```python
from build123d import *

# Parameters (mm, degrees)
SKETCH2_R                = 50.8
BOSS_EXTRUDE1_DEPTH      = 76.2
CUT_EXTRUDE4_START       = -6.35
SKETCH5_R                = 44.449999999999996
CUT_EXTRUDE4_DEPTH       = 63.5
CUT_EXTRUDE6_REACH       = 106.727
SKETCH14_R               = 7.62
BOSS_EXTRUDE4_REACH      = 170.227
BOSS_EXTRUDE4_END_RADIUS = 50.8
BOSS_EXTRUDE4_START      = 63.5
SKETCH17_W               = 52.06999999999999
SKETCH17_H               = 52.06999999999999
SKETCH15_W               = 11.430000000000003
SKETCH15_H               = 11.430000000000021
CUT_EXTRUDE7_DEPTH       = 112.44204771987995
CUT_EXTRUDE9_DEPTH       = 12.7
CUT_EXTRUDE10_DEPTH      = 112.44204771987995
CUT_EXTRUDE10_DEPTH_BACK = 112.44204771987995
SKETCH22_R               = 1.9049999999999998
SKETCH22_R_2             = 1.905
CUT_EXTRUDE11_DEPTH      = 6.35
CUT_EXTRUDE12_REACH      = 113.442
CUT_EXTRUDE12_END_RADIUS = 50.8


with BuildPart() as part:
    # Sketch2 → Boss-Extrude1 (new body)
    with BuildSketch(Plane(origin=(0, 0, 0), x_dir=(1, 0, 0), z_dir=(0, 1, 0))):
        with Locations(Location((0, 0, 0), (0, 0, 270))):
            Circle(SKETCH2_R)
    extrude(amount=-BOSS_EXTRUDE1_DEPTH)

    # Sketch5 → Cut-Extrude4 (cut)
    with BuildSketch(Plane(origin=(0, 0, 0), x_dir=(1, 0, 0), z_dir=(0, 1, 0)).offset(CUT_EXTRUDE4_START)):
        with Locations(Location((0, 0, 0), (0, 0, 270))):
            Circle(SKETCH5_R)
    extrude(amount=-CUT_EXTRUDE4_DEPTH, mode=Mode.SUBTRACT)

    # Sketch14 → Cut-Extrude6 (cut, up to next)
    with BuildSketch(Plane(origin=(0, 0, 0), x_dir=(1, 0, 0), z_dir=(0, 1, 0)), mode=Mode.PRIVATE) as cut_extrude6_sk1:
        with Locations(Location((0, 0, 0), (0, 0, 270))):
            Circle(SKETCH14_R)
    cut_extrude6_tool1 = extrude(cut_extrude6_sk1.sketch, amount=-CUT_EXTRUDE6_REACH, mode=Mode.PRIVATE) & part.part
    add(cut_extrude6_tool1.solids().sort_by_distance((0, 0, 0))[0], mode=Mode.SUBTRACT)

    # Boss-Extrude4: up to this cylinder (the profile starts outside it)
    boss_extrude4_end = Plane(origin=(0, -50.165, 0), z_dir=(0, 1, 0)) * Cylinder(BOSS_EXTRUDE4_END_RADIUS, 443.054, mode=Mode.PRIVATE)
    # Sketch17 → Boss-Extrude4 (add, up to the surface)
    with BuildSketch(Plane(origin=(0, 0, 0), x_dir=(0, 0, -1), z_dir=(1, 0, 0)).offset(BOSS_EXTRUDE4_START), mode=Mode.PRIVATE) as boss_extrude4_sk1:
        with Locations((0, -50.165000000000006)):
            Rectangle(SKETCH17_W, SKETCH17_H)
    boss_extrude4_tool1 = extrude(boss_extrude4_sk1.sketch, amount=-BOSS_EXTRUDE4_REACH, mode=Mode.PRIVATE) - boss_extrude4_end
    add(boss_extrude4_tool1.solids().sort_by_distance((63.5, -50.165, 0))[0])

    # Sketch15 → Cut-Extrude7 (cut, through all)
    with BuildSketch(Plane(origin=(0, 0, 0), x_dir=(0, 0, -1), z_dir=(1, 0, 0))):
        Polygon((8.890000000000002, -30.480000000000018), (8.890000000000004, -41.91000000000002), (20.320000000000007, -41.91000000000002), (20.320000000000004, -30.480000000000018), align=None)
        Polygon((8.890000000000004, -44.45000000000002), (8.890000000000004, -55.879999999999995), (20.32000000000001, -55.87999999999999), (20.320000000000004, -44.45000000000002), align=None)
        Polygon((8.890000000000004, -58.42000000000001), (8.890000000000006, -69.85000000000002), (20.320000000000007, -69.85000000000002), (20.320000000000004, -58.42000000000001), align=None)
        Polygon((-5.079999999999998, -30.480000000000018), (-5.0799999999999965, -41.91000000000002), (6.350000000000003, -41.91000000000002), (6.3500000000000005, -30.480000000000018), align=None)
        Polygon((-5.0799999999999965, -44.45000000000002), (-5.079999999999994, -55.879999999999995), (6.350000000000005, -55.879999999999995), (6.350000000000002, -44.45000000000002), align=None)
        Polygon((-5.079999999999994, -58.42000000000001), (-5.079999999999992, -69.85000000000002), (6.3500000000000085, -69.85000000000002), (6.350000000000005, -58.42000000000001), align=None)
        with Locations((-13.334999999999996, -64.13500000000002)):
            Rectangle(SKETCH15_W, SKETCH15_H)
        Polygon((-19.049999999999997, -44.45000000000002), (-19.049999999999997, -55.88), (-7.619999999999997, -55.88), (-7.620000000000001, -44.45000000000001), align=None)
        Polygon((-19.049999999999997, -30.480000000000018), (-19.049999999999997, -41.91000000000002), (-7.619999999999997, -41.91000000000002), (-7.619999999999999, -30.480000000000018), align=None)
    extrude(amount=CUT_EXTRUDE7_DEPTH, mode=Mode.SUBTRACT)

    # Sketch19 → Cut-Extrude9 (cut)
    with BuildSketch(Plane(origin=(63.5, 0, 0), x_dir=(0, 0, -1), z_dir=(1, 0, 0))):
        Polygon((-23.91833418, -26.24666582000001), (23.91833418, -26.24666582000001), (23.918334180000006, -74.08333418000001), (-23.918334179999995, -74.08333418000001), align=None)
        Polygon((-21.801668359999997, -28.36333164000001), (21.801668359999997, -28.36333164000001), (21.801668360000008, -71.96666836), (-21.80166835999999, -71.96666836), align=None, mode=Mode.SUBTRACT)
    extrude(amount=-CUT_EXTRUDE9_DEPTH, mode=Mode.SUBTRACT)

    # Sketch21 → Cut-Extrude10 (cut, two sides: drawn at the far end of the back side and taken through both)
    with BuildSketch(Plane.XY.offset(-CUT_EXTRUDE10_DEPTH_BACK)):
        Polygon((-50.8, -5.551e-14), (50.8, -5.551e-14), (50.8, -6.350000000000057), (-50.8, -6.350000000000056), align=None)
    extrude(amount=CUT_EXTRUDE10_DEPTH + CUT_EXTRUDE10_DEPTH_BACK, mode=Mode.SUBTRACT)

    # Sketch22 → Cut-Extrude11 (cut)
    with BuildSketch(Plane(origin=(-1.1e-16, -6.3500000000000565, 0), x_dir=(1, -2e-17, 0), z_dir=(2e-17, 1, 0))):
        with Locations(Location((-47.625, 0, 0), (0, 0, 180))):
            Circle(SKETCH22_R)
        with Locations(Location((-3.47e-15, 47.625, 0), (0, 0, 180))):
            Circle(SKETCH22_R_2)
        with Locations(Location((47.625, -2e-17, 0), (0, 0, 180))):
            Circle(SKETCH22_R)
        with Locations(Location((0, -47.625, 0), (0, 0, 180))):
            Circle(SKETCH22_R)
    extrude(amount=-CUT_EXTRUDE11_DEPTH, mode=Mode.SUBTRACT)

    # Sketch23 → Cut-Revolve2 (revolve, cut)
    with BuildSketch(Plane(origin=(-1.1e-16, -6.3500000000000565, 0), x_dir=(1, -2e-17, 0), z_dir=(2e-17, 1, 0))):
        with BuildLine():
            ThreePointArc((-35.92102448427656, 35.92102448427667), (-40.05586016064811, 31.243688431275256), (-43.58574874724786, 26.094491873607765))
            add(Edge.make_bspline(
                [(-43.58574874724785, 26.09449187360776), (-31.762489950913196, 24.642390713165252), (-27.206529454407143, 42.90040506855935)],
                knots=[0.20326690102876438, 0.20326690102876438, 0.20326690102876438, 2.6184475567908634, 2.6184475567908634, 2.6184475567908634], degree=2, weights=[1, 0.3552729019239298, 1]))
            ThreePointArc((-27.206529454407157, 42.90040506855938), (-31.756101065864836, 39.650851757491644), (-35.92102448427656, 35.921024484276664))
        make_face()
    cut_revolve2 = revolve(axis=Axis((-44.65936804956108, -6.350000000000056, -27.140852507845565), (0.6979571200610449, 0, -0.7161395524310135)), mode=Mode.SUBTRACT)

    # Mirror1: Cut-Revolve2 across plane
    add(cut_revolve2.mirror(Plane.XY), mode=Mode.SUBTRACT)

    # Mirror2: Cut-Revolve2 across plane
    add(cut_revolve2.mirror(Plane(origin=(0, 0, 0), x_dir=(0, 0, 1), z_dir=(1, 0, 0))), mode=Mode.SUBTRACT)

    # Mirror2 copy 1 sketch → Mirror2 copy 1 (revolve, cut)
    with BuildSketch(Plane(origin=(1.1e-16, -6.3500000000000565, 0), x_dir=(-1, -2e-17, 0), z_dir=(-2e-17, 1, 0))):
        with BuildLine():
            ThreePointArc((-35.92102448427656, 35.92102448427667), (-40.05586016064811, 31.243688431275256), (-43.58574874724786, 26.094491873607765))
            add(Edge.make_bspline(
                [(-43.58574874724785, 26.09449187360776), (-31.762489950913196, 24.642390713165252), (-27.206529454407143, 42.90040506855935)],
                knots=[0.20326690102876438, 0.20326690102876438, 0.20326690102876438, 2.6184475567908634, 2.6184475567908634, 2.6184475567908634], degree=2, weights=[1, 0.3552729019239298, 1]))
            ThreePointArc((-27.206529454407157, 42.90040506855938), (-31.756101065864836, 39.650851757491644), (-35.92102448427656, 35.921024484276664))
        make_face()
    revolve(axis=Axis((44.65936804956108, -6.350000000000056, 27.140852507845565), (-0.6979571200610449, 0, 0.7161395524310135)), mode=Mode.SUBTRACT)

    # Cut-Extrude12: up to this cylinder (the profile starts inside it)
    cut_extrude12_end = Plane(origin=(0, -19.049999999999997, 0), z_dir=(0, 1, 0)) * Cylinder(CUT_EXTRUDE12_END_RADIUS, 329.484, mode=Mode.PRIVATE)
    # Sketch24 → Cut-Extrude12 (cut, up to the surface)
    with BuildSketch(Plane(origin=(0, 0, 0), x_dir=(0, 0, -1), z_dir=(1, 0, 0)), mode=Mode.PRIVATE) as cut_extrude12_sk1:
        Polygon((19.05, -6.350000000000049), (-19.050000000000004, -6.350000000000054), (-19.05, -31.750000000000064), (19.050000000000008, -31.75000000000005), align=None)
    cut_extrude12_tool1 = extrude(cut_extrude12_sk1.sketch, amount=-CUT_EXTRUDE12_REACH, mode=Mode.PRIVATE) & cut_extrude12_end
    add(cut_extrude12_tool1.solids().sort_by_distance((0, -19.05, 0))[0], mode=Mode.SUBTRACT)


solid = part.part
```
Check sheet for the modelled part. Datum: model origin and axes. Units: mm. A direction names the side the tool comes from. Round coordinates to 2 decimals unless told otherwise and drop trailing zeros. Loops run counter-clockwise (first coordinate to the right, second up) from the corner with the lowest first, then second, coordinate; pieces in that order, holes last. Notation, with made-up numbers: (-37, 69) -> (5, 69) arc R15 ccw to (5, 92) -> close; hole circle Ø8 at (82.25, -11.75). An arc over 180 degrees is marked (long way). Write item = value, one per line. Start each with the question number.
1) Sectioned sample at B-B, the plane x = 0. Record the cut outline in (y, z).
2) Sectioned sample at A-A, the plane z = 0. State how many separate pieces and enclosed holes the cut face has, plus the area to 3 significant figures.
3) Sectioned sample at D-D, the plane y = -16.5. Record the cut outline in (x, z).
4) Set-up check for faces 4 (the flat face through (-44, -19, -19.05)), 5 (the cylindrical face through (0.413, -9.481, -49.485)), 6 (the flat face through (52, -64, 19.05)): record each of +Z, -Z, +X, -X, +Y, -Y from which the full face is reachable in a straight line by a thin tool's end or side.
5) Thickness scan on probe 1 along Y at (x, z) = (54, -21.5); probe 2 along Z at (x, y) = (0, -9.75); probe 3 along Z at (x, y) = (0, -35). Record the ranges inside material, lowest first.
6) Release check for a two-part mould opening along X. For faces 1 (the flat face through (63.5, -75, 2)), 2 (the flat face through (0, -12.7, -48)), 3 (the flat face through (51, -50, -20.32)) record: released by +X, released by -X, zero draft, split by the parting line, or undercut.
7) Gauge pin test, flat ends, axial feed: pin 1 Ø8 at (x, y) = (-14, -14) entering from -Z; pin 2 Ø3.5 at (x, y) = (50.5, -49) entering from -Z (3 decimals); pin 3 Ø1.5 at (x, y) = (-6.5, -31.5) entering from -Z. Record the tip position at first contact, or that the pin passes through.
Results are:
q1.outline = (-76.2, -50.8) -> (-6.35, -50.8) -> (-6.35, -49.53) -> (-12.7, -49.53) -> (-12.7, -45.72) -> (-6.35, -45.72) -> (-6.35, -44.45) -> (-69.85, -44.45) -> (-69.85, 44.45) -> (-6.35, 44.45) -> (-6.35, 45.72) -> (-12.7, 45.72) -> (-12.7, 49.53) -> (-6.35, 49.53) -> (-6.35, 50.8) -> (-76.2, 50.8) -> close
q2.separate_pieces = 4
q2.enclosed_holes = 0
q2.area = 1,220 mm^2
q3.outline = (-47.09, -19.05) arc R50.8 ccw (long way) to (-47.09, 19.05) -> (-40.16, 19.05) arc R44.45 cw (long way) to (-40.16, -19.05) -> close
q4.face_4 = -X, +Y
q4.face_5 = +Y
q4.face_6 = +X
q5.probe_1 = -76.2 to -74.08, -71.97 to -28.36, -26.25 to -24.13
q5.probe_2 = -50.8 to -49.53, -45.72 to -44.45, 44.45 to 45.72, 49.53 to 50.8
q5.probe_3 = -50.8 to -44.45, 44.45 to 50.8
q6.face_1 = released by +X
q6.face_2 = undercut
q6.face_3 = zero draft
q7.pin_1 = -49.81
q7.pin_2 = -26.035
q7.pin_3 = -50.47
